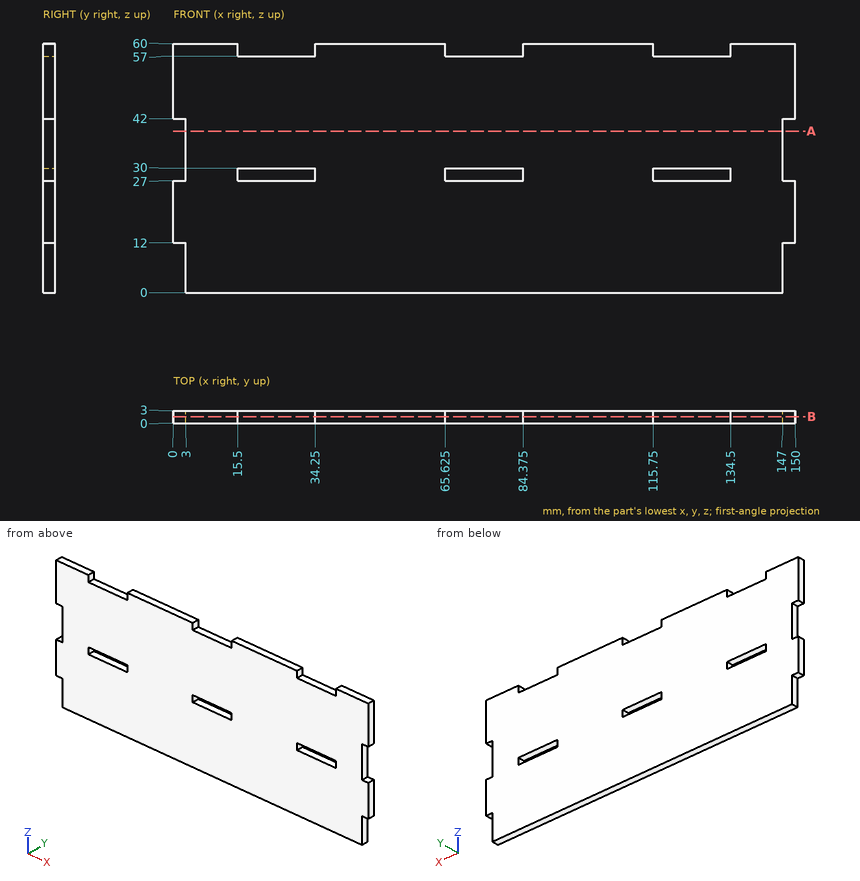
Input: dimensioned drawing with shaded views. Units: mm. Origin: part minimum x, y, z. Round coordinates to 2 decimals unless told otherwise and drop trailing zeros. Loops run counter-clockwise (first coordinate to the right, second up) from the corner with the lowest first, then second, coordinate; pieces in that order, holes last. Notation, with made-up numbers: (13.25, 88) -> (25.25, 88) arc R29 cw to (25.25, 118) -> close; hole circle Ø8 at (-15.5, 3.5). An arc over 180 degrees is marked (long way). One line per item, written item: value.
(1) Pin query (flat end, axial travel): pin 1 (0.9 mm diameter, centred on x = 129, y = 1.5, fed in from +Z); pin 2 (1 mm diameter, centred on y = 2.5, z = 31, fed in from -X); pin 3 (0.9 mm diameter, centred on y = 1, z = 28, fed in from +X). Return the tip coordinate at first contact, or that it passes through.
Geometry check:
pin 1: z = 57
pin 2: x = 3
pin 3: x = 147
(2) Section B-B (y = 1.55). Give the number of separate pieces and of enclosed holes in the cut face, plus the area to 3 significant figures.
Geometry check:
separate pieces: 1
enclosed holes: 3
area: 8,500 mm2
(3) Section A-A (z = 39). Return the cut outline in (x, y), plus the area to 3 significant figures.
Geometry check:
outline: (3, 0) -> (147, 0) -> (147, 3) -> (3, 3) -> close
area: 432 mm2
(4) Material intervals for line 1 (X direction, y = 0.25, z = 28) (3 decimals); line 2 (Z direction, x = 19.5, y = 1.95); line 3 (X direction, y = 1.35, z = 41), sorted ascending. Write a range as [from, to].
Geometry check:
line 1: [3, 15.5], [34.25, 65.625], [84.375, 115.75], [134.5, 147]
line 2: [0, 27], [30, 57]
line 3: [3, 147]
